```python
from build123d import *

# Parameters (mm, degrees)
SKETCH1_W                          = 25.4
SKETCH1_H                          = 38.1
BOSS_EXTRUDE1_DEPTH                = 15
SKETCH2_R                          = 11.51
CUT_EXTRUDE1_DEPTH                 = 2.38
SKETCH3_R                          = 4.95
CUT_EXTRUDE2_DEPTH                 = 2
SKETCH4_R                          = 0.625
CUT_EXTRUDE3_DEPTH                 = 48.005897502
SKETCH5_R                          = 1.22
CUT_EXTRUDE4_DEPTH                 = 49.184748624
SKETCH7_W                          = 5.7
SKETCH7_H                          = 12
CUT_EXTRUDE5_DEPTH                 = 49.184748624
SKETCH12_W                         = 5
SKETCH12_H                         = 15.45
BOSS_EXTRUDE2_DEPTH                = 14
SKETCH13_R                         = 1.59
SKETCH13_R_2                       = 1.7
CUT_EXTRUDE8_DEPTH                 = 7.5
TAP_DRILL_FOR_M2_5X0_45_TAP1_D     = 2.05
TAP_DRILL_FOR_M2_5X0_45_TAP1_DEPTH = 2.15
TAP_DRILL_FOR_M2_5X0_45_TAP1_TIP   = 0.615882135
SKETCH21_W                         = 5
SKETCH21_H                         = 13
CUT_EXTRUDE10_DEPTH                = 0.8
FILLET1_R                          = 0.79
SKETCH22_W                         = 8
SKETCH22_H                         = 10
BOSS_EXTRUDE3_DEPTH                = 5.7
SKETCH23_R                         = 2.02
CUT_EXTRUDE11_DEPTH                = 5.5
TAP_DRILL_FOR_10_32_TAP1_D         = 4.0386
TAP_DRILL_FOR_10_32_TAP1_DEPTH     = 5.5
TAP_DRILL_FOR_10_32_TAP1_TIP       = 1.213317848
SKETCH26_R                         = 0.625
CUT_EXTRUDE12_DEPTH                = 12.7
SKETCH27_R                         = 1.25
CUT_EXTRUDE13_DEPTH                = 8.22


with BuildPart() as part:
    # Sketch1 → Boss-Extrude1 (new body)
    with BuildSketch(Plane.XY):
        with Locations((12.7, 19.05)):
            Rectangle(SKETCH1_W, SKETCH1_H)
    extrude(amount=BOSS_EXTRUDE1_DEPTH)

    # Sketch2 → Cut-Extrude1 (cut)
    with BuildSketch(Plane.XY.offset(15)):
        with Locations((12.7, 19.05)):
            Circle(SKETCH2_R)
    extrude(amount=-CUT_EXTRUDE1_DEPTH, mode=Mode.SUBTRACT)

    # Sketch3 → Cut-Extrude2 (cut)
    with BuildSketch(Plane.XY.offset(12.62)):
        with Locations((12.7, 19.05)):
            Circle(SKETCH3_R)
    extrude(amount=-CUT_EXTRUDE2_DEPTH, mode=Mode.SUBTRACT)

    # Sketch4 → Cut-Extrude3 (cut, through all)
    with BuildSketch(Plane.XY.offset(10.62)):
        with Locations((12.7, 19.05)):
            Circle(SKETCH4_R)
    extrude(amount=-CUT_EXTRUDE3_DEPTH, mode=Mode.SUBTRACT)

    # Sketch5 → Cut-Extrude4 (cut, through all)
    with BuildSketch(Plane.XY.offset(15)):
        with Locations((2.92, 28.83)):
            Circle(SKETCH5_R)
        with Locations((22.48, 28.83)):
            Circle(SKETCH5_R)
        with Locations((22.48, 9.27)):
            Circle(SKETCH5_R)
        with Locations((2.92, 9.27)):
            Circle(SKETCH5_R)
    extrude(amount=-CUT_EXTRUDE4_DEPTH, mode=Mode.SUBTRACT)

    # Sketch7 → Cut-Extrude5 (cut, through all)
    with BuildSketch(Plane(origin=(0, 38.1, 0), x_dir=(1, 0, 0), z_dir=(0, 1, 0))):
        with Locations((2.85, -6)):
            Rectangle(SKETCH7_W, SKETCH7_H)
        with Locations((22.55, -6)):
            Rectangle(SKETCH7_W, SKETCH7_H)
    extrude(amount=-CUT_EXTRUDE5_DEPTH, mode=Mode.SUBTRACT)

    # Sketch12 → Boss-Extrude2 (add)
    with BuildSketch(Plane(origin=(19.7, 0, 0), x_dir=(0, 0, -1), z_dir=(1, 0, 0))):
        with Locations((-2.5, 45.825)):
            Rectangle(SKETCH12_W, SKETCH12_H)
        with Locations((-2.5, -7.725)):
            Rectangle(SKETCH12_W, SKETCH12_H)
    extrude(amount=-BOSS_EXTRUDE2_DEPTH)

    # Sketch13 → Cut-Extrude8 (cut)
    with BuildSketch(Plane.XY.offset(5)):
        with Locations((12.7, 48.55)):
            Circle(SKETCH13_R)
        with Locations((12.7, 42.55)):
            Circle(SKETCH13_R_2)
        with Locations((12.7, -4.45)):
            Circle(SKETCH13_R_2)
        with Locations((12.7, -10.45)):
            Circle(SKETCH13_R)
    extrude(amount=-CUT_EXTRUDE8_DEPTH, mode=Mode.SUBTRACT)

    # Tap Drill for M2.5x0.45 Tap1
    with Locations(Plane(origin=(19.7, 0, 0), x_dir=(0, 0, -1), z_dir=(1, 0, 0))):
        with Locations((-4.83, 16.46)):
            Hole(TAP_DRILL_FOR_M2_5X0_45_TAP1_D / 2, depth=TAP_DRILL_FOR_M2_5X0_45_TAP1_DEPTH)
            with Locations((0, 0, -(TAP_DRILL_FOR_M2_5X0_45_TAP1_DEPTH + TAP_DRILL_FOR_M2_5X0_45_TAP1_TIP / 2))):  # 118° drill point
                Cone(0, TAP_DRILL_FOR_M2_5X0_45_TAP1_D / 2, TAP_DRILL_FOR_M2_5X0_45_TAP1_TIP, mode=Mode.SUBTRACT)

    # Sketch21 → Cut-Extrude10 (cut)
    with BuildSketch(Plane(origin=(0, 0, 0), x_dir=(-1, 0, 0), z_dir=(0, 0, -1))):
        with Locations((-12.7, 19.05)):
            Rectangle(SKETCH21_W, SKETCH21_H)
    extrude(amount=-CUT_EXTRUDE10_DEPTH, mode=Mode.SUBTRACT)

    # Fillet1
    fillet1_edges = [part.edges().sort_by_distance(p)[0] for p in [
        (10.2, 25.55, 0.4),
        (10.2, 12.55, 0.4),
        (15.2, 12.55, 0.4),
        (15.2, 25.55, 0.4),
    ]]
    fillet(fillet1_edges, radius=FILLET1_R)

    # Sketch22 → Boss-Extrude3 (add)
    with BuildSketch(Plane.ZY.offset(-5.7)):
        with Locations((8, 19.05)):
            Rectangle(SKETCH22_W, SKETCH22_H)
    extrude(amount=BOSS_EXTRUDE3_DEPTH)

    # Sketch23 → Cut-Extrude11 (cut)
    with BuildSketch(Plane.ZY):
        with Locations((9, 19.05)):
            Circle(SKETCH23_R)
    extrude(amount=-CUT_EXTRUDE11_DEPTH, mode=Mode.SUBTRACT)

    # Tap Drill for #10-32 Tap1
    with Locations(Plane.ZY):
        with Locations((9, 19.05)):
            Hole(TAP_DRILL_FOR_10_32_TAP1_D / 2, depth=TAP_DRILL_FOR_10_32_TAP1_DEPTH)
            with Locations((0, 0, -(TAP_DRILL_FOR_10_32_TAP1_DEPTH + TAP_DRILL_FOR_10_32_TAP1_TIP / 2))):  # 118° drill point
                Cone(0, TAP_DRILL_FOR_10_32_TAP1_D / 2, TAP_DRILL_FOR_10_32_TAP1_TIP, mode=Mode.SUBTRACT)

    # Sketch26 → Cut-Extrude12 (cut)
    with BuildSketch(Plane.ZY):
        with Locations((9, 19.05)):
            Circle(SKETCH26_R)
    extrude(amount=-CUT_EXTRUDE12_DEPTH, mode=Mode.SUBTRACT)

    # Sketch27 → Cut-Extrude13 (cut)
    with BuildSketch(Plane.XY.offset(10.62)):
        with Locations((12.7, 19.05)):
            Circle(SKETCH27_R)
    extrude(amount=-CUT_EXTRUDE13_DEPTH, mode=Mode.SUBTRACT)


solid = part.part
```
Source: CAD feature listing. Evaluate the final solid. Frame: model axes, mm. A direction names the side the tool comes from. Give positions to 0.01 mm unless a question says otherwise; leave off trailing zeros. Write each loop counter-clockwise with the first axis right and the second up, starting at its lowest first coordinate (ties: lowest second). Pieces come first, ordered by that corner, then holes.
1. Section query B-B (x = 2.92). Return the cut outline in (y, z).
2. Material intervals for line 1 along Y through (x, z) = (12.7, 1.4) (3 decimals); line 2 along X through (y, z) = (-10.5, 2.75); line 3 along Y through (x, z) = (12.7, 13.7), sorted ascending.
3. Pull-direction query (Z, two-part tool) for faces 6 (the face through (14, 18, 10.62)), 7 (the face through (3, 19, 4)), 8 (the face through (17.04, 16.29, 4.87)); classes: +Z half, -Z half, draft (parallel to the pull), parting line (faces both ways), or undercut.
4. Section query D-D (y = 9.27). Return the cut outline in (x, z).
5. Section query A-A (y = -10.45). Return the cut outline in (x, z), then the cut area to 3 significant figures.
6. Access query for faces 1 (the face through (13, -8, 5)), 2 (the face through (14, 19, 0.8)), 3 (the face through (19.7, 20, 5)), 4 (the face through (7.755, 19.268, 11.634)), 5 (the face through (3, 31, 12)). Directions: +Z, -Z, +X, -X, +Y, -Y. A direction counts if a zero-diameter tool reaches every point of the face in a straight line with its end or side. Return the directions, or none.
7. First-contact query: pin 1 (1.5 mm diameter, centred on y = 24.5, z = 11, fed in from -X); pin 2 (13 mm diameter, centred on x = 12.7, y = 19.05, fed in from +Z); pin 3 (6.5 mm diameter, centred on x = 2.5, z = 8, fed in from -Y); pin 4 (3 mm diameter, centred on x = 11.5, y = 17.5, fed in from +Z). Flat tips, straight axial feed; report the tip coordinate or a pass-through.
Output values:
1. outline: (0, 12) - (8.05, 12) - (8.05, 15) - (0, 15) - close; (10.49, 12) - (14.05, 12) - (14.05, 4) - (24.05, 4) - (24.05, 12) - (27.61, 12) - (27.61, 15) - (25.12, 15) - (25.12, 12.62) - (12.98, 12.62) - (12.98, 15) - (10.49, 15) - close; (30.05, 12) - (38.1, 12) - (38.1, 15) - (30.05, 15) - close; hole circle Ø4.04 at (19.05, 9)
2. line 1: y = -15.45 to -12.04, -8.86 to -6.15, -2.75 to 18.425, 19.675 to 40.85, 44.25 to 46.96, 50.14 to 53.55
2. line 2: x = 5.7 to 11.11, 14.29 to 19.7
2. line 3: y = 0 to 7.54, 30.56 to 38.1
3. face 6: +Z half
3. face 7: -Z half
3. face 8: undercut
4. outline: (0, 12) - (1.7, 12) - (1.7, 15) - (0, 15) - close; (4.14, 12) - (5.7, 12) - (5.7, 0) - (19.7, 0) - (19.7, 12) - (21.26, 12) - (21.26, 15) - (18.77, 15) - (18.77, 12.62) - (6.63, 12.62) - (6.63, 15) - (4.14, 15) - close; (23.7, 12) - (25.4, 12) - (25.4, 15) - (23.7, 15) - close
5. outline: (5.7, 0) - (11.11, 0) - (11.11, 5) - (5.7, 5) - close; (14.29, 0) - (19.7, 0) - (19.7, 5) - (14.29, 5) - close
5. area: 54.1 mm2
6. face 1: +Z, +X, -X, -Y
6. face 2: -Z
6. face 3: -Z, +X, +Y, -Y
6. face 4: +Z
6. face 5: -Z, -X, +Y
7. pin 1: stops at x = 0
7. pin 2: stops at z = 12.62
7. pin 3: stops at y = 0
7. pin 4: stops at z = 10.62
